Design review of the part built by this model. Coordinates are the model's own, in mm. A direction names the side the tool comes from. Round coordinates to 2 decimals unless told otherwise and drop trailing zeros. Write each loop counter-clockwise with the first axis right and the second up, starting at its lowest first coordinate (ties: lowest second). Pieces come first, ordered by that corner, then holes. Notation, with made-up numbers: (47.25, -8) -> (106.25, -8) arc R35 ccw to (106.25, 25) -> close; hole circle Ø9 at (-18, -39). An arc over 180 degrees is marked (long way). Write item = value, one per line. Start each with the question number.
Item 1: Add section C-C, the plane z = 5.25. State the section outline as (x, y) points, then the cut area to 3 significant figures.
Item 2: Add section B-B, the plane y = -1.5. State the section outline as (x, z) points (1 decimal), then the cut area to 3 significant figures.
Item 3: Mouldability with a two-part tool opening along X and no side actions: class faces 1 (the cylindrical face through (10.99, -7.73, 0.71)), 2 (the flat face through (-12.7, -7.1, 8.4)), 3 (the flat face through (12.7, -7, 3)) as released by +X, released by -X, zero draft, split by the parting line, or undercut.
Item 4: Machinability: for faces 4 (the cylindrical face through (0.246, -9.836, 8.982)), 5 (the flat face through (0, -1, 7.937)), which of the approach directions +Z, -Z, +X, -X, +Y, -Y give a long, thin tool a straight path to every point of the face, cutting with its end or side? Answer none if there is none.
Item 5: Add section D-D, the plane x = -4.5. State how many separate pieces and enclosed holes the cut face has, then the cut area to 3 significant figures.
Item 6: For pin 1 Ø3 at (x, z) = (-9, -1) entering from +Y; pin 2 Ø14.5 at (x, y) = (0, 5.56) entering from -Z; pin 3 Ø4 at (x, z) = (4.5, -4) entering from -Y, all flat-tipped, find the tip position at first contact; note any pin that passes through.
Item 7: Add section A-A, the plane z = 1.5. State the section outline as (x, y) points, then the cut area to 3 significant figures.
Item 8: To check wall thickness, follow L1, parallel to Z at x = 6.25, y = 0.75 (1 decimal); L2, parallel to Y at x = 0, z = 8.8; L3, parallel to Y at x = 0, z = 9.1. State the ranges of each line that lie inside material, in increasing order.
from build123d import *

# Parameters (mm, degrees)
F0_W      = 25.4
F0_H      = 19.05
F1_DEPTH  = 12.7
F3_DEPTH  = 19.051
F4_DEPTH  = 17.4625
F5_R      = 1.27
F6_R      = 1.905
F7_R      = 2.3495
F8_DEPTH  = 25.0151169265
F10_R     = 5.08
F9_R      = 5.5626
F11_DEPTH = 19.051


with BuildPart() as f1:
    # F0 (on Front) → F1 (new body, symmetric)
    with BuildSketch(Plane.XZ):
        Rectangle(F0_W, F0_H)
    extrude(amount=F1_DEPTH, both=True)

    # F2 (on face) → F3 (cut, through all)
    with BuildSketch(Plane(origin=(0, 0, -9.525), x_dir=(1, 0, 0), z_dir=(0, 0, -1))):
        Polygon((12.7, 12.7), (-12.7, 12.7), (12.7, 8.22129469), align=None)
    extrude(amount=-F3_DEPTH, mode=Mode.SUBTRACT)

    # F2 (on face) → F4 (cut)
    with BuildSketch(Plane(origin=(0, 0, -9.525), x_dir=(1, 0, 0), z_dir=(0, 0, -1))):
        Polygon((12.7, 6.6093049436), (-12.7, 11.0880102536), (-12.7, -12.7), (12.7, -12.7), align=None)
    extrude(amount=-F4_DEPTH, mode=Mode.SUBTRACT)

    # F5
    f5_edges = [f1.edges().sort_by_distance(p)[0] for p in [
        (0, -8.848658, 7.9375),
    ]]
    fillet(f5_edges, radius=F5_R)

    # F6
    f6_edges = [f1.edges().sort_by_distance(p)[0] for p in [
        (0, -10.460647, 9.525),
    ]]
    fillet(f6_edges, radius=F6_R)

    # F7 (on face) → F8 (cut, through all)
    with BuildSketch(Plane(origin=(1.7888760521, -10.1452202319, 0), x_dir=(0.984807753, 0.1736481777, 0), z_dir=(0.1736481777, -0.984807753, 0))):
        with Locations((7.239, 0)):
            Circle(F7_R)
        with Locations((-7.239, 0)):
            Circle(F7_R)
    extrude(amount=-F8_DEPTH, mode=Mode.SUBTRACT)

    # F10
    f10_edges = [f1.edges().sort_by_distance(p)[0] for p in [
        (12.7, 12.7, 8.73125),
        (-12.7, 12.7, 8.73125),
    ]]
    fillet(f10_edges, radius=F10_R)

    # F9 (on face) → F11 (cut, through all)
    with BuildSketch(Plane.XY.offset(9.525)):
        with Locations((0, 5.5626)):
            Circle(F9_R)
    extrude(amount=-F11_DEPTH, mode=Mode.SUBTRACT)


solid = f1.part
Result set:
q1.outline = (-12.7, -12.7) -> (12.7, -8.22) -> (12.7, -6.61) -> (-12.7, -11.09) -> close
q1.area = 40.9 mm²
q2.outline = (-12.7, 7.9) -> (12.7, 7.9) -> (12.7, 9.5) -> (-12.7, 9.5) -> close
q2.area = 40.3 mm²
q3.face_1 = undercut
q3.face_2 = released by -X
q3.face_3 = released by +X
q4.face_4 = +Z, +X, -Y
q4.face_5 = -Z, -X, +Y
q5.separate_pieces = 3
q5.enclosed_holes = 0
q5.area = 48.5 mm²
q6.pin_1 = -10.18
q6.pin_2 = 7.94
q6.pin_3 = -10.02
q7.outline = (-12.7, -12.7) -> (-7.12, -11.72) -> (-7.4, -10.15) -> (-12.7, -11.09) -> close; (-3.83, -9.52) -> (-3.56, -11.09) -> (7.14, -9.2) -> (6.86, -7.64) -> close; (10.42, -7.01) -> (10.7, -8.57) -> (12.7, -8.22) -> (12.7, -6.61) -> close
q7.area = 29.5 mm²
q8.L1 = 7.9 to 9.5
q8.L2 = -10.04 to 0, 11.13 to 12.7
q8.L3 = -9.74 to 0, 11.13 to 12.7
